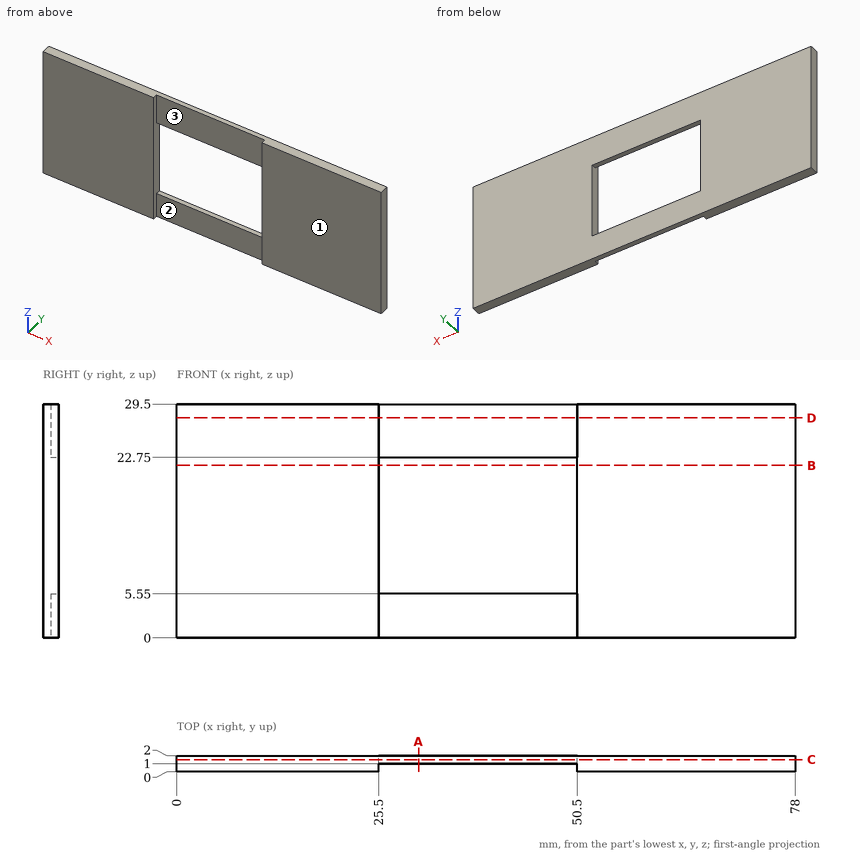
Study the drawing (mm; zero at the part's minimum x, y, z) and answer. Give positions to 0.01 mm unless a question says otherwise; leave off trailing zeros. Order: outer loops, then holes, each group sorted by start corner. A loop starts at its lowest first (then second) coordinate and runs counter-clockwise, first axis right, second up. Notation, with made-up numbers: (83, 27) - (111, 27) arc R17 cw to (111, 35) - close; hole circle Ø5 at (-38.75, 66.25). An arc over 180 degrees is marked (long way). Use one line per item in the form item = value. Start each with the question number.
(1) The mould has two halves that part along X. Classify the marked faces 1, 2 and 3: released by +X, released by -X, zero draft, split by the parting line, or undercut.
(2) A cutting plane is placed at A-A, the plane x = 30.5. Write down the section's boundary in (y, z).
(3) A cutting plane is placed at D-D, the plane z = 27.75. Write down the section's boundary in (x, y).
(4) A cutting plane is placed at B-B, the plane z = 21.75. Write down the section's boundary in (x, y), then the cut area to 3 significant figures.
(5) Consider line 1 (X direction, y = 0.45, z = 9); line 2 (Z direction, x = 37.5, y = 1.75); line 3 (Y direction, x = 29.5, z = 25). Determine where each line is inside the solid, lowest interval first. Write a range as from..to.
(6) A flat-ended cylindrical pin translates along its axis: pin 1 Ø1.7 at (x, z) = (43, 4) entering from -Y. Find the tip coordinate at first contact, or state that the pin passes through.
(7) A cutting plane is placed at C-C, the plane y = 1.5. Write down the section's boundary in (x, z), then the cut area to 3 significant figures.
Ans:
q1.face_1 = zero draft
q1.face_2 = undercut
q1.face_3 = undercut
q2.outline = (1, 0) - (2, 0) - (2, 5.55) - (1, 5.55) - close; (1, 22.75) - (2, 22.75) - (2, 29.5) - (1, 29.5) - close
q3.outline = (0, 0) - (25.5, 0) - (25.5, 1) - (50.5, 1) - (50.5, 0) - (78, 0) - (78, 2) - (0, 2) - close
q4.outline = (0, 0) - (25.5, 0) - (25.5, 2) - (0, 2) - close; (50.5, 0) - (78, 0) - (78, 2) - (50.5, 2) - close
q4.area = 106 mm^2
q5.line_1 = 0..25.5, 50.5..78
q5.line_2 = 0..5.55, 22.75..29.5
q5.line_3 = 1..2
q6.pin_1 = 1
q7.outline = (0, 0) - (78, 0) - (78, 29.5) - (0, 29.5) - close; hole (25.5, 5.55) - (50.5, 5.55) - (50.5, 22.75) - (25.5, 22.75) - close
q7.area = 1,870 mm^2
